Design review of the part built by this model. Coordinates are the model's own, in mm. Give positions to 0.01 mm unless a question says otherwise; leave off trailing zeros. Loops run counter-clockwise (first coordinate to the right, second up) from the corner with the lowest first, then second, coordinate; pieces in that order, holes last. Notation, with made-up numbers: (63, -4) -> (99, -4) arc R14 ccw to (99, 22) -> close; hole circle Ø3 at (-13, 9). An arc over 180 degrees is marked (long way). Use CSV: the item, a comma, the result in double quotes. Start each with the question number.
Item 1: Clearance check with flat-ended pins moving along their axes: pin 1 (1.5 mm diameter, centred on x = 2823, y = 1109, fed in from -Z); pin 2 (7 mm diameter, centred on x = 2819.6, y = 1133.24, fed in from +Z); pin 3 (1.3 mm diameter, centred on y = 1132, z = 0.5, fed in from +X); pin 4 (1.8 mm diameter, centred on y = 1088, z = -15.5, fed in from -X) (3 decimals). State where each tip first meets the part, or that it passes through.
Item 2: We need section C-C (x = 2767.5). State the section outline as (y, z) points.
Item 3: We need section A-A (z = -17). State the section outline as (x, y) points, plus the area to 3 significant figures.
Item 4: We need section B-B (x = 2795.5). State the section outline as (y, z) points, plus the area to 3 significant figures.
Item 5: Wall thickness on line 1 along Z through (x, y) = (2794, 1149.5); line 2 along Y through (x, z) = (2840.5, -1.5); line 3 along Y through (x, z) = (2778.5, -11): over which ranges is each line inside the solid? List them lowest first. Write a range as from..to.
Item 6: We need section D-D (y = 1101.5). State the section outline as (x, z) points, plus the area to 3 significant figures.
Item 7: The part is to be moulded in two halves that separate along Y. For faces 1 (the face through (2767.507, 1150.02, 0.587)), 2 (the face through (2786.584, 1105.038, 0.587)), 3 (the face through (2831.925, 1087, -12)), 4 (the face through (2796.636, 1112.373, 0.587)), say which applies: +Y half, -Y half, draft (parallel to the pull), parting line (faces both ways), or undercut.
from build123d import *

# Parameters (mm, degrees)
CROQUIS1_R              = 4.430496459
CROQUIS1_R_2            = 2.021537648
CROQUIS1_R_3            = 3.175
CROQUIS1_R_4            = 2.776444448
CROQUIS1_R_5            = 2.106249137
SALIENTE_EXTRUIR1_DEPTH = 1.19
CROQUIS4_W              = 27.78454451
CROQUIS4_H              = 1.19
SALIENTE_EXTRUIR2_DEPTH = 33.19
REDONDEO2_R             = 5


with BuildPart() as part:
    # Croquis1 → Saliente-Extruir1 (new body)
    with BuildSketch(Plane.XY):
        with BuildLine():
            Line((2788.515923591, 1163.062896503), (2845.320282862, 1163.062896503))
            ThreePointArc((2845.320282862, 1163.062896503), (2854.380265752, 1158.219977336), (2857.861371877, 1148.554623946))
            Line((2857.861371877, 1148.554623946), (2857.861371877, 1105.884683704))
            Line((2857.861371877, 1105.884683704), (2859.709564321, 1099.969499723))
            Line((2859.709564321, 1099.969499723), (2859.709564321, 1086.668463787))
            Line((2859.709564321, 1086.668463787), (2831.925019811, 1086.668463787))
            Line((2831.925019811, 1086.668463787), (2831.925019811, 1090.237043102))
            ThreePointArc((2831.925019811, 1090.237043102), (2830.339855276, 1092.909707682), (2827.46732338, 1094.094799688))
            Line((2827.46732338, 1094.094799688), (2781.073788136, 1094.094799688))
            ThreePointArc((2781.073788136, 1094.094799688), (2777.943377157, 1096.10205762), (2777.077273901, 1099.718467781))
            Line((2777.077273901, 1099.718467781), (2777.077273901, 1139.357764533))
            ThreePointArc((2777.077273901, 1139.357764533), (2776.16191908, 1141.931561181), (2774.31245647, 1143.941981956))
            Line((2774.31245647, 1143.941981956), (2760.508490421, 1156.27030536))
            Line((2760.508490421, 1156.27030536), (2756.869619555, 1168.884626052))
            ThreePointArc((2756.869619555, 1168.884626052), (2756.826740412, 1171.777711215), (2757.827792947, 1174.492425601))
            Line((2757.827792947, 1174.492425601), (2758.788780948, 1178.67068333))
            Line((2758.788780948, 1178.67068333), (2784.893128388, 1172.66675387))
            Line((2784.893128388, 1172.66675387), (2784.19129322, 1169.615260811))
            ThreePointArc((2784.19129322, 1169.615260811), (2784.56217485, 1165.156713392), (2788.515923591, 1163.062896503))
        make_face()
        with Locations((2819.601763615, 1133.235396685)):
            Circle(CROQUIS1_R, mode=Mode.SUBTRACT)
        with Locations((2790.727223865, 1121.638053324)):
            Circle(CROQUIS1_R_2, mode=Mode.SUBTRACT)
        with Locations((2783.65094449, 1147.375154376)):
            Circle(CROQUIS1_R_3, mode=Mode.SUBTRACT)
        with Locations((2793.607825607, 1111.419307874)):
            Circle(CROQUIS1_R_3, mode=Mode.SUBTRACT)
        with Locations((2783.65094449, 1106.253651095)):
            Circle(CROQUIS1_R_3, mode=Mode.SUBTRACT)
        with Locations((2842.913546585, 1132.266044758)):
            Circle(CROQUIS1_R_4, mode=Mode.SUBTRACT)
        with Locations((2843.009293559, 1122.033928625)):
            Circle(CROQUIS1_R_5, mode=Mode.SUBTRACT)
        with Locations((2843.009293559, 1114.670632569)):
            Circle(CROQUIS1_R_3, mode=Mode.SUBTRACT)
    extrude(amount=SALIENTE_EXTRUIR1_DEPTH)

    # Croquis4 → Saliente-Extruir2 (add)
    with BuildSketch(Plane.XY.offset(1.19)):
        with Locations((2845.817292066, 1087.263463787)):
            Rectangle(CROQUIS4_W, CROQUIS4_H)
        Polygon((2784.893128388, 1172.66675387), (2784.626395606, 1171.507032515), (2758.522048166, 1177.510961974), (2758.788780948, 1178.67068333), align=None)
    extrude(amount=-SALIENTE_EXTRUIR2_DEPTH)

    # Redondeo2
    redondeo2_edges = [part.edges().sort_by_distance(p)[0] for p in [
        (2784.759761997, 1172.086893193, -32),
        (2758.655414557, 1178.090822652, -32),
        (2831.925019811, 1087.263463787, -32),
        (2859.709564321, 1087.263463787, -32),
    ]]
    fillet(redondeo2_edges, radius=REDONDEO2_R)


solid = part.part
Results found:
1,pin 1,"z = 0"
1,pin 2,"through"
1,pin 3,"x = 2857.86"
1,pin 4,"x = 2831.925"
2,outline,"(1150.03, 0) -> (1175.45, 0) -> (1175.45, -32) -> (1176.67, -32) -> (1176.67, 1.19) -> (1150.03, 1.19) -> close"
3,outline,"(2758.52, 1177.51) -> (2784.63, 1171.51) -> (2784.89, 1172.67) -> (2758.79, 1178.67) -> close; (2831.93, 1086.67) -> (2859.71, 1086.67) -> (2859.71, 1087.86) -> (2831.93, 1087.86) -> close"
3,area,"64.9 mm²"
4,outline,"(1094.09, 0) -> (1108.87, 0) -> (1108.87, 1.19) -> (1094.09, 1.19) -> close; (1113.97, 0) -> (1163.06, 0) -> (1163.06, 1.19) -> (1113.97, 1.19) -> close"
4,area,"76.0 mm²"
5,line 1,"0..1.19"
5,line 2,"1086.67..1087.86"
5,line 3,"1172.92..1174.14"
6,outline,"(2777.08, 0) -> (2859.23, 0) -> (2859.23, 1.19) -> (2777.08, 1.19) -> close"
6,area,"97.8 mm²"
7,face 1,"-Y half"
7,face 2,"undercut"
7,face 3,"draft"
7,face 4,"undercut"
